Read the model definition and answer for the solid it produces. Units are mm, in the model's axes. A direction names the side the tool comes from. Coordinates: 2 decimals unless noted, no trailing zeros. Loops run counter-clockwise (first coordinate to the right, second up) from the corner with the lowest first, then second, coordinate; pieces in that order, holes last. Notation, with made-up numbers: M 60,10.25 L 116,10.25 A22 ccw 116,25.25 Z; hole C 26,42 d9. An arc over 180 degrees is marked long. One line per item, written item: value. Start each with the question number.
1. The part is cut by section C-C (z = 0.8). State how many separate pieces and enclosed holes the cut face has, then the cut area to 3 significant figures.
2. The part is cut by section B-B (x = 45.5). Write down the section's boundary in (y, z), then the cut area to 3 significant figures.
3. Flat-ended cylindrical pins translate along their axes: pin 1 (3.5 mm diameter, centred on x = -156.79, y = -18.19, fed in from -Z); pin 2 (0.9 mm diameter, centred on x = -48, z = 1.5, fed in from +Y); pin 3 (1.5 mm diameter, centred on y = 95, z = 2, fed in from -X); pin 4 (1.5 mm diameter, centred on x = -49.5, z = 1.5, fed in from -Y). Find the tip coordinate at first contact, or state that the pin passes through.
4. Consider probe 1 along X at (y, z) = (194, 0.2); probe 2 along X at (y, z) = (62, 0.3); probe 3 along Y at (x, z) = (-73, 1.55). Determine where each line is inside the solid, lowest interval first.
5. Determine the mould class of faces 5 (the face through (-14.467, -16.24, 1.479)), 6 (the face through (51.86, 49.13, 1.48)), 7 (the face through (-89.117, 189.852, 1.479)), 8 (the face through (-154.84, 49.48, 1.48)) for opening direction Y: +Y half, -Y half, draft (parallel to the pull), parting line (faces both ways), or undercut.
6. The part is cut by section A-A (y = 54). Write down the section's boundary in (x, z), then the cut area to 3 significant figures.
7. For faces 1 (the face through (-155.44, 124.48, 1.48)), 2 (the face through (-89.47, -16.85, 1.48)), 3 (the face through (51.25, 124.13, 1.48)), 4 (the face through (-14.117, 190.459, 1.479)), determine the directions among +Z, -Z, +X, -X, +Y, -Y from which every point of the face is accessible in a straight line to the end or side of a thin tool.
```python
from build123d import *

# Parameters (mm, degrees)
F0_R     = 50
F1_DEPTH = 3
F2_D     = 4.4
F3_D     = 4


with BuildPart() as f1:
    # F0 (on Top) → F1 (new body)
    with BuildSketch(Plane.XY):
        with BuildLine():
            Line((-101.7921956682, 211.8060733306), (-171.7921956682, 211.8060733306))
            ThreePointArc((-171.7921956682, 211.8060733306), (-175.3277295741, 210.3416072366), (-176.7921956682, 206.8060733306))
            Line((-176.7921956682, 206.8060733306), (-176.7921956682, 136.8060733306))
            Line((-176.7921956682, 136.8060733306), (-133.490925479, 111.8060733306))
            Line((-133.490925479, 111.8060733306), (-133.490925479, 61.8060733306))
            Line((-133.490925479, 61.8060733306), (-176.7921956682, 36.8060733306))
            Line((-176.7921956682, 36.8060733306), (-176.7921956682, -33.1939266694))
            ThreePointArc((-176.7921956682, -33.1939266694), (-175.3277295741, -36.7294605753), (-171.7921956682, -38.1939266694))
            Line((-171.7921956682, -38.1939266694), (-101.7921956682, -38.1939266694))
            Line((-101.7921956682, -38.1939266694), (-76.7921956682, 5.1073435198))
            Line((-76.7921956682, 5.1073435198), (-26.7921956682, 5.1073435198))
            Line((-26.7921956682, 5.1073435198), (-1.7921956682, -38.1939266694))
            Line((-1.7921956682, -38.1939266694), (68.2078043318, -38.1939266694))
            ThreePointArc((68.2078043318, -38.1939266694), (71.7433382377, -36.7294605753), (73.2078043318, -33.1939266694))
            Line((73.2078043318, -33.1939266694), (73.2078043318, 36.8060733306))
            Line((73.2078043318, 36.8060733306), (29.9065341426, 61.8060733306))
            Line((29.9065341426, 61.8060733306), (29.9065341426, 111.8060733306))
            Line((29.9065341426, 111.8060733306), (73.2078043318, 136.8060733306))
            Line((73.2078043318, 136.8060733306), (73.2078043318, 206.8060733306))
            ThreePointArc((73.2078043318, 206.8060733306), (71.7433382377, 210.3416072366), (68.2078043318, 211.8060733306))
            Line((68.2078043318, 211.8060733306), (-1.7921956682, 211.8060733306))
            Line((-1.7921956682, 211.8060733306), (-26.7921956682, 168.5048031414))
            Line((-26.7921956682, 168.5048031414), (-76.7921956682, 168.5048031414))
            Line((-76.7921956682, 168.5048031414), (-101.7921956682, 211.8060733306))
        make_face()
        with Locations((-51.7921956682, 86.8060733306)):
            Circle(F0_R, mode=Mode.SUBTRACT)
    extrude(amount=F1_DEPTH)

    # F2 (through all)
    with Locations(Plane(origin=(0, 0, 0), x_dir=(1, 0, 0), z_dir=(0, 0, -1))):
        with Locations((-111.7921956682, -146.8060733306), (-111.7921956682, -26.8060733306), (8.2078043318, -26.8060733306), (8.2078043318, -146.8060733306)):
            Hole(F2_D / 2)

    # F3 (through all)
    with Locations(Plane(origin=(0, 0, 0), x_dir=(1, 0, 0), z_dir=(0, 0, -1))):
        with Locations((-156.7921956682, -191.8060733306), (-156.7921956682, 18.1939266694), (53.2078043318, 18.1939266694), (53.2078043318, -191.8060733306)):
            Hole(F3_D / 2)


solid = f1.part
```
Answer block:
1. separate pieces: 1
1. enclosed holes: 9
1. area: 41,500 mm2
2. outline: M -38.19,0 L 52.8,0 L 52.8,3 L -38.19,3 Z; M 120.81,0 L 211.81,0 L 211.81,3 L 120.81,3 Z
2. area: 546 mm2
3. pin 1: passes through
3. pin 2: stops at y = 168.5
3. pin 3: stops at x = -133.49
3. pin 4: stops at y = 5.11
4. probe 1: x = -176.79 to -91.51, -12.07 to 73.21
4. probe 2: x = -133.49 to -95.2, -8.38 to 29.91
4. probe 3: y = 5.11 to 41.53, 132.09 to 168.5
5. face 5: -Y half
5. face 6: undercut
5. face 7: +Y half
5. face 8: undercut
6. outline: M -147.01,0 L -89.52,0 L -89.52,3 L -147.01,3 Z; M -14.06,0 L 43.43,0 L 43.43,3 L -14.06,3 Z
6. area: 345 mm2
7. face 1: +Z, -Z, -X
7. face 2: +Z, -Z, -Y
7. face 3: +Z, -Z, +X
7. face 4: +Z, -Z, +Y
